Design review of the part built by this model. Coordinates are the model's own, in mm. Give positions to 0.01 mm unless a question says otherwise; leave off trailing zeros. Write each loop counter-clockwise with the first axis right and the second up, starting at its lowest first coordinate (ties: lowest second). Pieces come first, ordered by that corner, then holes. Notation, with made-up numbers: (52, -10.75) -> (59, -10.75) arc R31 ccw to (59, 17.25) -> close; hole circle Ø1 at (86, -3.75). An arc over 180 degrees is marked (long way). Answer as a JSON object with one key per item and string values.
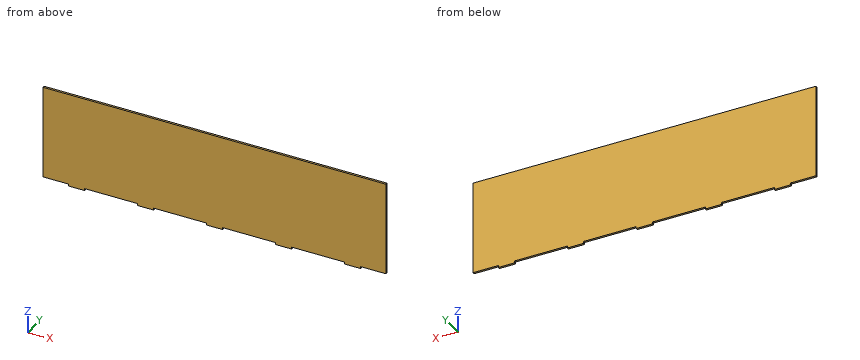
```python
from build123d import *

# Parameters (mm, degrees)
SKETCH1_W           = 534.99766
SKETCH1_H           = 147.69846
BOSS_EXTRUDE1_DEPTH = 3.175
SKETCH2_W           = 25.4
SKETCH2_H           = 3.175
BOSS_EXTRUDE2_DEPTH = 3.175


with BuildPart() as part:
    # Sketch1 → Boss-Extrude1 (new body)
    with BuildSketch(Plane(origin=(0, 0, 0), x_dir=(1, 0, 0), z_dir=(0, 1, 0))):
        with Locations((267.49883, 73.84923)):
            Rectangle(SKETCH1_W, SKETCH1_H)
    extrude(amount=BOSS_EXTRUDE1_DEPTH)

    # Sketch2 → Boss-Extrude2 (add)
    with BuildSketch(Plane(origin=(0, 0, -147.69846), x_dir=(-1, 0, 0), z_dir=(0, 0, -1))):
        with Locations((-482.77145, 1.5875)):
            Rectangle(SKETCH2_W, SKETCH2_H)
        with Locations((-375.14403, 1.5875)):
            Rectangle(SKETCH2_W, SKETCH2_H)
        with Locations((-267.665260384, 1.5875)):
            Rectangle(SKETCH2_W, SKETCH2_H)
        with Locations((-159.888954488, 1.5875)):
            Rectangle(SKETCH2_W, SKETCH2_H)
        with Locations((-52.098109833, 1.5875)):
            Rectangle(SKETCH2_W, SKETCH2_H)
    extrude(amount=BOSS_EXTRUDE2_DEPTH)


solid = part.part
```
(1) Clearance check with flat-ended pins moving along their axes: pin 1 (1.6 mm diameter, centred on y = 2, z = -149, fed in from -X); pin 2 (1 mm diameter, centred on y = 1.5, z = -149, fed in from +X); pin 3 (1 mm diameter, centred on x = 198.5, y = 2, fed in from -Z). State where each tip first meets the part, or that it passes through.
Here are the results:
{"pin 1": "stops at x = 39.4", "pin 2": "stops at x = 495.47", "pin 3": "stops at z = -147.7"}
(2) For line 1 along Z through (x, y) = (120.5, 2.75), list the stretches that pass through material, from the lowest coordinate up.
Here are the results:
{"line 1": "z = -147.7 to 0"}
(3) We need section B-B, the plane x = 401. State the section outline as (y, z) points (3 decimals), then the cut area to 3 significant figures.
Here are the results:
{"outline": "(0, -147.698) -> (3.175, -147.698) -> (3.175, 0) -> (0, 0) -> close", "area": "469 mm²"}
(4) We need section A-A, the plane y = 2.55. State the section outline as (x, z) points.
Here are the results:
{"outline": "(0, -147.7) -> (39.4, -147.7) -> (39.4, -150.87) -> (64.8, -150.87) -> (64.8, -147.7) -> (147.19, -147.7) -> (147.19, -150.87) -> (172.59, -150.87) -> (172.59, -147.7) -> (254.97, -147.7) -> (254.97, -150.87) -> (280.37, -150.87) -> (280.37, -147.7) -> (362.44, -147.7) -> (362.44, -150.87) -> (387.84, -150.87) -> (387.84, -147.7) -> (470.07, -147.7) -> (470.07, -150.87) -> (495.47, -150.87) -> (495.47, -147.7) -> (535, -147.7) -> (535, 0) -> (0, 0) -> close"}
